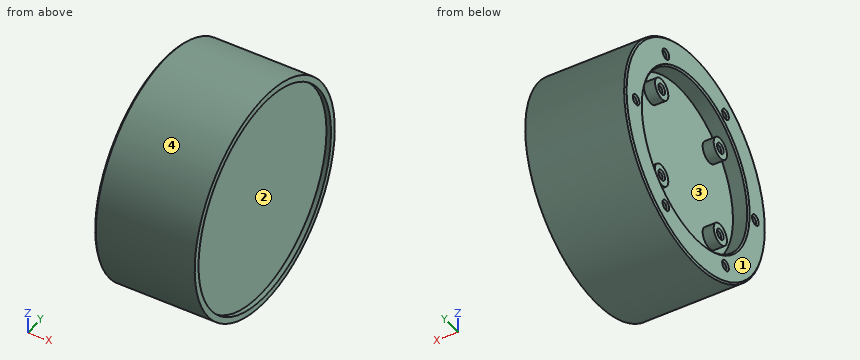
from build123d import *

# Parameters (mm, degrees)
SKETCH1_R                    = 37
BOSS_EXTRUDE1_DEPTH          = 16.83
SKETCH2_R                    = 1.25
CUT_EXTRUDE1_DEPTH           = 6.7
CHAMFER1_SIZE                = 0.5
CIRPATTERN1_COUNT            = 6
CHAMFER1_OF_CIRPATTERN1_SIZE = 0.5
SKETCH3_R                    = 28
CUT_EXTRUDE2_DEPTH           = 5.2
SKETCH4_R                    = 3.5
BOSS_EXTRUDE2_DEPTH          = 3.65
SKETCH5_R                    = 1.25
CUT_EXTRUDE3_DEPTH           = 5.15
CHAMFER2_SIZE                = 0.5
CHAMFER3_SIZE                = 0.5
SKETCH6_R                    = 35
CUT_EXTRUDE4_DEPTH           = 2
SKETCH7_R                    = 37
SKETCH7_R_2                  = 35
CUT_EXTRUDE5_DEPTH           = 0.5


with BuildPart() as part:
    # Sketch1 → Boss-Extrude1 (new, symmetric)
    with BuildSketch(Plane(origin=(0, 0, 0), x_dir=(0, 0, -1), z_dir=(1, 0, 0))):
        Circle(SKETCH1_R)
    extrude(amount=BOSS_EXTRUDE1_DEPTH, both=True)

    # Sketch2 → Cut-Extrude1 (cut)
    with BuildSketch(Plane.ZY.offset(16.83)):
        with Locations((0, 31.5)):
            Circle(SKETCH2_R)
    cut_extrude1 = extrude(amount=-CUT_EXTRUDE1_DEPTH, mode=Mode.SUBTRACT)

    # Chamfer1
    chamfer1_edges = [part.edges().sort_by_distance(p)[0] for p in [
        (-16.83, 31.5, -1.25),
    ]]
    chamfer(chamfer1_edges, length=CHAMFER1_SIZE)

    # CirPattern1: Cut-Extrude1 ×6 about axis
    cirpattern1_axis = Axis((0, 0, 0), (1, 0, 0))
    for i in range(1, CIRPATTERN1_COUNT):
        add(cut_extrude1.rotate(cirpattern1_axis, i * 360 / CIRPATTERN1_COUNT), mode=Mode.SUBTRACT)

    # Chamfer1 of CirPattern1
    chamfer1_of_cirpattern1_edges = [part.edges().sort_by_distance(p)[0] for p in [
        (-16.83, 16.832531755, 26.654800219),
        (-16.83, -14.667468245, 27.904800219),
        (-16.83, -31.5, 1.25),
        (-16.83, -16.832531755, -26.654800219),
        (-16.83, 14.667468245, -27.904800219),
    ]]
    chamfer(chamfer1_of_cirpattern1_edges, length=CHAMFER1_OF_CIRPATTERN1_SIZE)

    # Sketch3 → Cut-Extrude2 (cut)
    with BuildSketch(Plane.ZY.offset(16.83)):
        Circle(SKETCH3_R)
    extrude(amount=-CUT_EXTRUDE2_DEPTH, mode=Mode.SUBTRACT)

    # Sketch4 → Boss-Extrude2 (add)
    with BuildSketch(Plane.ZY.offset(11.63)):
        with Locations((15.5, 15.5)):
            Circle(SKETCH4_R)
        with Locations((-15.5, 15.5)):
            Circle(SKETCH4_R)
        with Locations((-15.5, -15.5)):
            Circle(SKETCH4_R)
        with Locations((15.5, -15.5)):
            Circle(SKETCH4_R)
    extrude(amount=BOSS_EXTRUDE2_DEPTH)

    # Sketch5 → Cut-Extrude3 (cut)
    with BuildSketch(Plane.ZY.offset(15.28)):
        with Locations((-15.5, 15.5)):
            Circle(SKETCH5_R)
        with Locations((15.5, 15.5)):
            Circle(SKETCH5_R)
        with Locations((15.5, -15.5)):
            Circle(SKETCH5_R)
        with Locations((-15.5, -15.5)):
            Circle(SKETCH5_R)
    extrude(amount=-CUT_EXTRUDE3_DEPTH, mode=Mode.SUBTRACT)

    # Chamfer2
    chamfer2_edges = [part.edges().sort_by_distance(p)[0] for p in [
        (-16.83, 0, 37),
        (-16.83, 0, -28),
    ]]
    chamfer(chamfer2_edges, length=CHAMFER2_SIZE)

    # Chamfer3
    chamfer3_edges = [part.edges().sort_by_distance(p)[0] for p in [
        (-15.28, -15.5, -16.75),
        (-15.28, -15.5, 14.25),
        (-15.28, 15.5, 14.25),
        (-15.28, 15.5, -16.75),
    ]]
    chamfer(chamfer3_edges, length=CHAMFER3_SIZE)

    # Sketch6 → Cut-Extrude4 (cut)
    with BuildSketch(Plane(origin=(16.83, 0, 0), x_dir=(0, 0, -1), z_dir=(1, 0, 0))):
        Circle(SKETCH6_R)
    extrude(amount=-CUT_EXTRUDE4_DEPTH, mode=Mode.SUBTRACT)

    # Sketch7 → Cut-Extrude5 (cut)
    with BuildSketch(Plane(origin=(16.83, 0, 0), x_dir=(0, 0, -1), z_dir=(1, 0, 0))):
        Circle(SKETCH7_R)
        Circle(SKETCH7_R_2, mode=Mode.SUBTRACT)
    extrude(amount=-CUT_EXTRUDE5_DEPTH, mode=Mode.SUBTRACT)


solid = part.part
Design review of the part built by this model. Coordinates are the model's own, in mm. Face numbers are marked on the shaded views. Give positions to 0.01 mm unless a question says otherwise; leave off trailing zeros. Loops run counter-clockwise (first coordinate to the right, second up) from the corner with the lowest first, then second, coordinate; pieces in that order, holes last. Notation, with made-up numbers: M 78,32 L 89,32 A8 cw 89,36 Z; hole C -6.75,-4.75 d7. An arc over 180 degrees is marked long. Write item = value, one per line.
Q1. Insertion check: pin 1 (2 mm diameter, centred on y = 14.5, z = -16.5, fed in from -X); pin 2 (1.5 mm diameter, centred on y = 15.5, z = -15.5, fed in from -X); pin 3 (5 mm diameter, centred on x = -5, y = 22.5, fed in from +Z). Each pin has a flat end and moves straight along its axis. Give the tip position at first contact, or say it passes through.
Output values:
pin_1 = -15.28
pin_2 = -10.13
pin_3 = 31.13
Q2. We need section B-B (x = 3). Give the boundary of the cut face in (y, z), plus the area to 3 significant figures.
Output values:
outline = C 0,0 d74
area = 4,300 mm^2
Q3. To check wall thickness, follow line 1 (Y direction, x = -13.7, z = 0); line 2 (Y direction, x = 9, z = 22); line 3 (X direction, y = 6, z = -29.5). State the ranges of each line that lie inside material, in increasing order. Write a range as [from, to].
Output values:
line_1 = [-37, -32.75], [-30.25, -28], [28, 30.25], [32.75, 37]
line_2 = [-29.75, 29.75]
line_3 = [-16.83, 14.83]
Q4. Draft analysis for pull direction Y (two halves, no side actions). For the marked faces 1, 2, 3 and 4, state which applies: +Y half, -Y half, draft (parallel to the pull), parting line (faces both ways), or undercut.
Output values:
face_1 = draft
face_2 = undercut
face_3 = undercut
face_4 = parting line
Q5. We need section A-A (y = 0). Give the boundary of the cut face in (x, z).
Output values:
outline = M -16.83,-36.5 L -16.33,-37 L 16.33,-37 L 16.33,-35 L 14.83,-35 L 14.83,35 L 16.33,35 L 16.33,37 L -16.33,37 L -16.83,36.5 L -16.83,28.5 L -16.33,28 L -11.63,28 L -11.63,-28 L -16.33,-28 L -16.83,-28.5 Z
